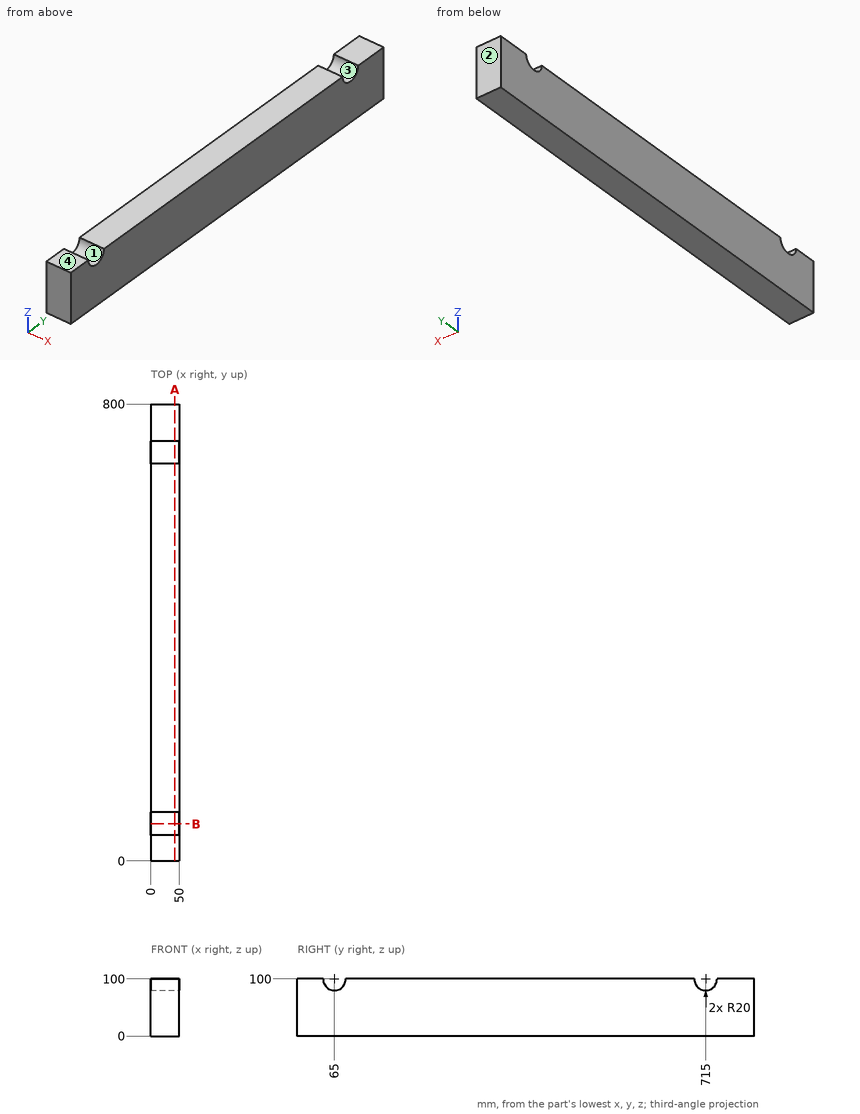
For this review, use the dimensioned drawing (mm, ordinates from the lowest corner) and the shaded views. Coordinates: 2 decimals unless noted, no trailing zeros. Write each loop counter-clockwise with the first axis right and the second up, starting at its lowest first coordinate (ties: lowest second). Pieces come first, ordered by that corner, then holes. Notation, with made-up numbers: (55.5, -1.75) -> (95.5, -1.75) arc R26 ccw to (95.5, 28.25) -> close; hole circle Ø11 at (-31, 19.5). An arc over 180 degrees is marked (long way). Put each result on its own line as item: value.
Q1. Wall thickness on L1, parallel to Z at x = 37, y = 717: over which ranges is the line inside the solid? List them lowest first.
From the geometry:
L1: z = 0 to 80.1
Q2. The part is to be moulded in two halves that separate along Y. For the marked faces 1, 2, 3 and 4, say which applies: +Y half, -Y half, draft (parallel to the pull), parting line (faces both ways), or undercut.
From the geometry:
face 1: undercut
face 2: +Y half
face 3: undercut
face 4: draft
Q3. Take a section at A-A, the plane x = 42. State the section outline as (y, z) points, then the cut area to 3 significant figures.
From the geometry:
outline: (0, 0) -> (800, 0) -> (800, 100) -> (735, 100) arc R20 cw to (695, 100) -> (85, 100) arc R20 cw to (45, 100) -> (0, 100) -> close
area: 78,700 mm2
Q4. Take a section at B-B, the plane y = 65. State the section outline as (x, z) points, then the cut area to 3 significant figures.
From the geometry:
outline: (0, 0) -> (50, 0) -> (50, 80) -> (0, 80) -> close
area: 4,000 mm2
